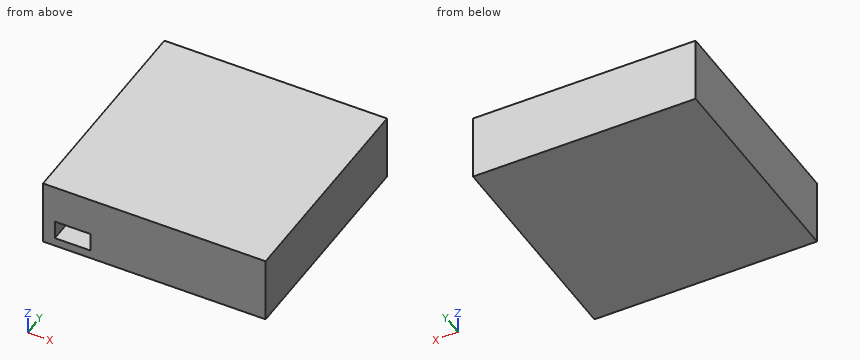
```python
from build123d import *

# Parameters (mm, degrees)
SCHIZZO1_W                   = 41.2
SCHIZZO1_H                   = 41.2
ESTRUSIONE_ESTRUSIONE1_DEPTH = 12.3
SCHIZZO2_W                   = 6.6
SCHIZZO2_H                   = 3.5
TAGLIO_ESTRUSIONE1_DEPTH     = 42
SCHIZZO3_W                   = 6.6
SCHIZZO3_H                   = 2.261378951
ESTRUSIONE_ESTRUSIONE2_DEPTH = 5


with BuildPart() as part:
    # Schizzo1 → Estrusione-Estrusione1 (new body)
    with BuildSketch(Plane.XY):
        with Locations((20.6, 20.6)):
            Rectangle(SCHIZZO1_W, SCHIZZO1_H)
    extrude(amount=ESTRUSIONE_ESTRUSIONE1_DEPTH)

    # Schizzo2 → Taglio-Estrusione1 (cut)
    with BuildSketch(Plane(origin=(0, 41.2, 0), x_dir=(1, 0, 0), z_dir=(0, 1, 0))):
        with Locations((5.5, -3.35)):
            Rectangle(SCHIZZO2_W, SCHIZZO2_H)
    extrude(amount=-TAGLIO_ESTRUSIONE1_DEPTH, mode=Mode.SUBTRACT)

    # Schizzo3 → Estrusione-Estrusione2 (add)
    with BuildSketch(Plane(origin=(0, 0, 5.1), x_dir=(-1, 0, 0), z_dir=(0, 0, -1))):
        with Locations((-5.5, 40.069310525)):
            Rectangle(SCHIZZO3_W, SCHIZZO3_H)
    extrude(amount=ESTRUSIONE_ESTRUSIONE2_DEPTH)


solid = part.part
```
Design review of the part built by this model. Coordinates are the model's own, in mm. Coordinates: 2 decimals unless noted, no trailing zeros. Order: outer loops, then holes, each group sorted by start corner. A loop starts at its lowest first (then second) coordinate and runs counter-clockwise, first axis right, second up. Notation, with made-up numbers: (74.25, 65) - (83.25, 65) arc R21 ccw to (83.25, 79) - close; hole circle Ø4 at (-9, 4.5). An arc over 180 degrees is marked (long way). Answer in a Markdown table with one row per item.
(1) Consider section B-B on x = 5.5. State the section outline as (y, z) points, plus the area to 3 significant figures.
Checked values:
| item | result |
|---|---|
| outline | (0, 0) - (41.2, 0) - (41.2, 12.3) - (0, 12.3) - (0, 5.1) - (38.94, 5.1) - (38.94, 1.6) - (0, 1.6) - close |
| area | 370 mm^2 |
(2) Consider section A-A on y = 33.5. State the section outline as (x, z) points, plus the area to 3 significant figures.
Checked values:
| item | result |
|---|---|
| outline | (0, 0) - (41.2, 0) - (41.2, 12.3) - (0, 12.3) - close; hole (2.2, 1.6) - (8.8, 1.6) - (8.8, 5.1) - (2.2, 5.1) - close |
| area | 484 mm^2 |
(3) Clearance check with a flat-ended pin moving along its axis: pin 1 (1.7 mm diameter, centred on x = 7, z = 4, fed in from -Y). State where the tip first meets the part, or that it passes through.
Checked values:
| item | result |
|---|---|
| pin 1 | y = 38.94 |
(4) Wall thickness on line 1 along X through (y, z) = (21.5, 4.5); line 2 along Z through (x, y) = (4, 9.5); line 3 along Y through (x, z) = (6, 2): over which ranges is each line inside the solid? List them lowest first. Write a range as from..to.
Checked values:
| item | result |
|---|---|
| line 1 | 0..2.2, 8.8..41.2 |
| line 2 | 0..1.6, 5.1..12.3 |
| line 3 | 38.94..41.2 |
(5) Consider section C-C on z = 2.25. State the section outline as (x, y) points.
Checked values:
| item | result |
|---|---|
| outline | (0, 0) - (2.2, 0) - (2.2, 38.94) - (8.8, 38.94) - (8.8, 0) - (41.2, 0) - (41.2, 41.2) - (0, 41.2) - close |
